Source: CAD feature listing. Evaluate the final solid. Frame: model axes, mm. A direction names the side the tool comes from. Round coordinates to 2 decimals unless told otherwise and drop trailing zeros. Order: outer loops, then holes, each group sorted by start corner. A loop starts at its lowest first (then second) coordinate and runs counter-clockwise, first axis right, second up. Notation, with made-up numbers: (6.25, -9.5) - (31.25, -9.5) arc R19 ccw to (31.25, 15.5) - close; hole circle Ø4 at (55, -6.75). An arc over 180 degrees is marked (long way). Return JSON: item names as keys, results as strings. Group by question number.
1) Section B-B, the plane x = -52. Return loops of the section in (y, z).
2) Contact query for flat-ended pins moving along their axis: P1, Ø5, axis at x = 28, z = 6, coming from the -Y side; P2, Ø1, axis at y = -46, z = 31, coming from the -X side; P3, Ø1.5, axis at y = -45.5, z = -3.5, coming from the -X side. Output: stop coordinate, or through.
3) Section A-A, the plane z = -41. Return loops of the section in (x, y).
4) Ray query, line 1 (X direction, y = 20, z = -56); line 2 (X direction, y = -1, z = -53); line 3 (X direction, y = -47.5, z = 20.5). Return the intervals inside material, ascending. Write a range as from..to.
5) Mould query, pull axis X, two halves, no side actions, for faces 4 (the cylindrical face through (-44.506, 38.376, -56.972)), 5 (the flat face through (-1, 1, 69.85)), 6 (the flat face through (-28, -27, 6.35)). Classes: pulls with the +X half, pulls with the -X half, needs draft (parallel to the pull), parting line crosses it, or undercut.
6) Access query for faces 1 (the flat face through (6.347, -30, -38)), 2 (the flat face through (-1, 1, -69.85)), 3 (the flat face through (-33, -7.356, 39)). Directions: +Z, -Z, +X, -X, +Y, -Y. A direction counts if a zero-diameter tool reaches every point of the face in a straight line with its end or side. Return the directions, or none.
7) Section D-D, the plane z = 1.5. Return loops of the section in (x, y).
8) Section C-C, the plane y = 53.5. Return loops of the section in (x, z), plus the area to 3 significant figures.
```python
from build123d import *

# Parameters (mm, degrees)
F0_R     = 67.0773206954
F1_DEPTH = 69.85
F2_DEPTH = 6.35
F3_DEPTH = 44.45


# Not quite as in the source:
# - a feature names something its author has since deleted; it is built from what else it names


with BuildPart() as f1:
    # F0 (on Top) → F1 (new body, symmetric)
    with BuildSketch(Plane.XY):
        Circle(F0_R)
        with BuildLine():
            ThreePointArc((58.4782874441, 5.8071771637), (58.6939681668, 2.9071480599), (58.7659204727, 0))
            ThreePointArc((58.7659204727, 0), (43.7402884604, -39.2456440183), (6.3470844528, -58.4221527159))
            ThreePointArc((6.3470844528, -58.4221527159), (-0.5649559649, -58.7632047608), (-7.469161507, -58.2893217956))
            ThreePointArc((-7.469161507, -58.2893217956), (-41.5941780551, -41.5133443718), (-58.3037411026, -7.3557584547))
            ThreePointArc((-58.3037411026, -7.3557584547), (-58.6502618149, -3.6851320266), (-58.7659204727, 0))
            ThreePointArc((-58.7659204727, 0), (-44.1155616542, 38.8233258357), (-7.469161507, 58.2893217956))
            ThreePointArc((-7.469161507, 58.2893217956), (-0.5649559649, 58.7632047608), (6.3470844528, 58.4221527159))
            ThreePointArc((6.3470844528, 58.4221527159), (41.745252706, 41.3614226729), (58.4782874441, 5.8071771637))
        make_face(mode=Mode.SUBTRACT)
        with BuildLine():
            ThreePointArc((-7.469161507, -58.2893217956), (-0.5649559649, -58.7632047608), (6.3470844528, -58.4221527159))
            Line((6.3470844528, -58.4221527159), (6.3470844528, 0))
            Line((6.3470844528, 0), (6.3470844528, 5.8071771637))
            Line((6.3470844528, 5.8071771637), (6.3470844528, 58.4221527159))
            ThreePointArc((6.3470844528, 58.4221527159), (-0.5649559649, 58.7632047608), (-7.469161507, 58.2893217956))
            Line((-7.469161507, 58.2893217956), (-7.469161507, 0))
            Line((-7.469161507, 0), (-7.469161507, -7.3557584547))
            Line((-7.469161507, -7.3557584547), (-7.469161507, -58.2893217956))
        make_face()
        with BuildLine():
            Line((6.3470844528, 0), (58.7659204727, 0))
            ThreePointArc((58.7659204727, 0), (58.6939681668, 2.9071480599), (58.4782874441, 5.8071771637))
            Line((58.4782874441, 5.8071771637), (6.3470844528, 5.8071771637))
            Line((6.3470844528, 5.8071771637), (6.3470844528, 0))
        make_face()
        with BuildLine():
            ThreePointArc((-58.7659204727, 0), (-58.6502618149, -3.6851320266), (-58.3037411026, -7.3557584547))
            Line((-58.3037411026, -7.3557584547), (-7.469161507, -7.3557584547))
            Line((-7.469161507, -7.3557584547), (-7.469161507, 0))
            Line((-7.469161507, 0), (-58.7659204727, 0))
        make_face()
    extrude(amount=F1_DEPTH, both=True)

    # F0 (on Top) → F2 (join, symmetric)
    with BuildSketch(Plane.XY):
        with BuildLine():
            ThreePointArc((-58.7659204727, 0), (-58.6502618149, -3.6851320266), (-58.3037411026, -7.3557584547))
            Line((-58.3037411026, -7.3557584547), (-7.469161507, -7.3557584547))
            Line((-7.469161507, -7.3557584547), (-7.469161507, 0))
            Line((-7.469161507, 0), (-58.7659204727, 0))
        make_face()
        with BuildLine():
            Line((6.3470844528, 5.8071771637), (58.4782874441, 5.8071771637))
            ThreePointArc((58.4782874441, 5.8071771637), (41.745252706, 41.3614226729), (6.3470844528, 58.4221527159))
            Line((6.3470844528, 58.4221527159), (6.3470844528, 5.8071771637))
        make_face()
        with BuildLine():
            ThreePointArc((6.3470844528, -58.4221527159), (43.7402884604, -39.2456440183), (58.7659204727, 0))
            Line((58.7659204727, 0), (6.3470844528, 0))
            Line((6.3470844528, 0), (6.3470844528, -58.4221527159))
        make_face()
        with BuildLine():
            ThreePointArc((-58.3037411026, -7.3557584547), (-41.5941780551, -41.5133443718), (-7.469161507, -58.2893217956))
            Line((-7.469161507, -58.2893217956), (-7.469161507, -7.3557584547))
            Line((-7.469161507, -7.3557584547), (-58.3037411026, -7.3557584547))
        make_face()
    extrude(amount=F2_DEPTH, both=True)

    # F0 (on Top) → F3 (join, symmetric)
    with BuildSketch(Plane.XY):
        with BuildLine():
            Line((-7.469161507, 0), (-7.469161507, 58.2893217956))
            ThreePointArc((-7.469161507, 58.2893217956), (-44.1155616542, 38.8233258357), (-58.7659204727, 0))
            Line((-58.7659204727, 0), (-7.469161507, 0))
        make_face()
    extrude(amount=F3_DEPTH, both=True)


solid = f1.part
```
Geometry check:
{
 "1": {"outline": "(-42.37, -69.85) - (-27.38, -69.85) - (-27.38, -6.35) - (-7.36, -6.35) - (-7.36, -69.85) - (0, -69.85) - (0, -44.45) - (27.38, -44.45) - (27.38, -69.85) - (42.37, -69.85) - (42.37, 69.85) - (27.38, 69.85) - (27.38, 44.45) - (0, 44.45) - (0, 69.85) - (-7.36, 69.85) - (-7.36, 6.35) - (-27.38, 6.35) - (-27.38, 69.85) - (-42.37, 69.85) - close"},
 "2": {"P1": "y = -62.04", "P2": "x = -49.29", "P3": "x = -49.97"},
 "3": {"outline": "circle Ø134.15 at (0, 0); hole (-58.3, -7.36) arc R58.77 ccw to (-7.47, -58.29) - (-7.47, -7.36) - close; hole (6.35, -58.42) arc R58.77 ccw to (58.77, 0) - (6.35, 0) - close; hole (6.35, 5.81) - (58.48, 5.81) arc R58.77 ccw to (6.35, 58.42) - close"},
 "4": {"line 1": "-64.03..-55.26, -7.47..6.35, 55.26..64.03", "line 2": "-67.07..6.35, 58.76..67.07", "line 3": "-47.36..-34.6, -7.47..6.35, 34.6..47.36"},
 "5": {"face 4": "undercut", "face 5": "needs draft", "face 6": "undercut"},
 "6": {"face 1": "-Z", "face 2": "-Z, +X, -X, +Y, -Y", "face 3": "+Z"},
 "7": {"outline": "circle Ø134.15 at (0, 0)"},
 "8": {"outline": "(-40.46, -69.85) - (-24.31, -69.85) - (-24.31, -44.45) - (-7.47, -44.45) - (-7.47, -69.85) - (6.35, -69.85) - (6.35, -6.35) - (24.31, -6.35) - (24.31, -69.85) - (40.46, -69.85) - (40.46, 69.85) - (24.31, 69.85) - (24.31, 6.35) - (6.35, 6.35) - (6.35, 69.85) - (-7.47, 69.85) - (-7.47, 44.45) - (-24.31, 44.45) - (-24.31, 69.85) - (-40.46, 69.85) - close", "area": "8,170 mm2"}
}
